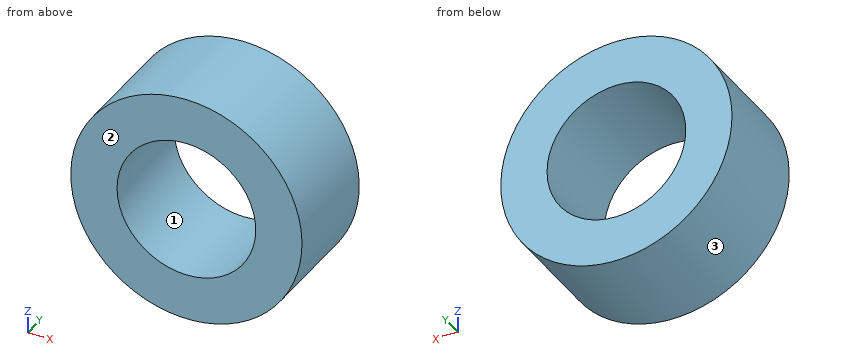
```python
from build123d import *

# Parameters (mm, degrees)
SKETCH1_W            = 11
SKETCH1_H            = 11
BOSS_EXTRUDE1_DEPTH  = 5
M6_CLEARANCE_HOLE1_D = 6.6
SKETCH4_OUTSIDE_W    = 16.268
SKETCH4_OUTSIDE_H    = 16.268
SKETCH4_OUTSIDE_R    = 5.5
CUT_EXTRUDE1_DEPTH   = 10.246621004


with BuildPart() as part:
    # Sketch1 → Boss-Extrude1 (new body)
    with BuildSketch(Plane(origin=(0, 0, 0), x_dir=(1, 0, 0), z_dir=(0, 1, 0))):
        Rectangle(SKETCH1_W, SKETCH1_H)
    extrude(amount=BOSS_EXTRUDE1_DEPTH)

    # M6 Clearance Hole1 (through all)
    with Locations(Plane(origin=(0, 5, 0), x_dir=(1, 0, 0), z_dir=(0, 1, 0))):
        with Locations((0, 0)):
            Hole(M6_CLEARANCE_HOLE1_D / 2)

    # Sketch4 outside → Cut-Extrude1 (cut, through all)
    with BuildSketch(Plane(origin=(0, 5, 0), x_dir=(1, 0, 0), z_dir=(0, 1, 0))):
        Rectangle(SKETCH4_OUTSIDE_W, SKETCH4_OUTSIDE_H)
        with Locations(Location((0, 0, 0), (0, 0, 270))):
            Circle(SKETCH4_OUTSIDE_R, mode=Mode.SUBTRACT)
    extrude(amount=-CUT_EXTRUDE1_DEPTH, mode=Mode.SUBTRACT)


solid = part.part
```
Geometry: final body of the model. Coordinates: model frame, mm. Face numbers are marked on the shaded views. Round coordinates to 2 decimals unless told otherwise and drop trailing zeros. Write each loop counter-clockwise with the first axis right and the second up, starting at its lowest first coordinate (ties: lowest second). Pieces come first, ordered by that corner, then holes. Notation, with made-up numbers: (27, 31.5) -> (47, 31.5) arc R25 cw to (47, 64.5) -> close; hole circle Ø4 at (75.5, 20). An arc over 180 degrees is marked (long way). Return JSON: item names as keys, results as strings.
Q1. Section C-C on y = 2.3. Return the cut outline in (x, z).
From the geometry:
{"outline": "circle Ø11 at (0, 0); hole circle Ø6.6 at (0, 0)"}
Q2. Mould query, pull axis Z, two halves, no side actions, for the marked faces 1, 2 and 3. Classes: +Z half, -Z half, draft (parallel to the pull), parting line (faces both ways), or undercut.
From the geometry:
{"face 1": "undercut", "face 2": "draft", "face 3": "parting line"}
Q3. Ray query, line 1 (Z direction, x = 0, y = 3.4); line 2 (X direction, y = 4.7, z = -3); line 3 (Z direction, x = 1, y = 2). Return the intervals inside material, ascending.
From the geometry:
{"line 1": "-5.5 to -3.3, 3.3 to 5.5", "line 2": "-4.61 to -1.37, 1.37 to 4.61", "line 3": "-5.41 to -3.14, 3.14 to 5.41"}
Q4. Section D-D on z = 4.5. Return the cut outline in (x, y).
From the geometry:
{"outline": "(-3.16, 0) -> (3.16, 0) -> (3.16, 5) -> (-3.16, 5) -> close"}
Q5. Section A-A on z = 0. Return the cut outline in (x, y), and give its area (3 significant figures).
From the geometry:
{"outline": "(-5.5, 0) -> (-3.3, 0) -> (-3.3, 5) -> (-5.5, 5) -> close; (3.3, 0) -> (5.5, 0) -> (5.5, 5) -> (3.3, 5) -> close", "area": "22.0 mm2"}
Q6. Section B-B on x = 0. Return the cut outline in (y, z).
From the geometry:
{"outline": "(0, -5.5) -> (5, -5.5) -> (5, -3.3) -> (0, -3.3) -> close; (0, 3.3) -> (5, 3.3) -> (5, 5.5) -> (0, 5.5) -> close"}
Q7. First-contact query: pin 1 Ø4 at (x, z) = (-3.5, -1) entering from -Y; pin 2 Ø3 at (x, y) = (3.5, 2.5) entering from -Z. Flat tips, straight axial feed; report the tip coordinate or a pass-through.
From the geometry:
{"pin 1": "y = 0", "pin 2": "z = -5.12"}
